from build123d import *

# Parameters (mm, degrees)
SKETCH1_W           = 130
SKETCH1_H           = 82
BOSS_EXTRUDE1_DEPTH = 4
SKETCH2_W           = 40
SKETCH2_H           = 10
CUT_EXTRUDE1_DEPTH  = 24
BOSS_EXTRUDE2_DEPTH = 4
SKETCH4_W           = 10
SKETCH4_H           = 10
BOSS_EXTRUDE3_DEPTH = 24
SKETCH5_R           = 2
CUT_EXTRUDE2_DEPTH  = 151


with BuildPart() as part:
    # Sketch1 → Boss-Extrude1 (new body)
    with BuildSketch(Plane(origin=(0, 0, 0), x_dir=(1, 0, 0), z_dir=(0, 1, 0))):
        Rectangle(SKETCH1_W, SKETCH1_H)
    extrude(amount=BOSS_EXTRUDE1_DEPTH)

    # Sketch2 → Cut-Extrude1 (cut)
    with BuildSketch(Plane(origin=(0, 4, 0), x_dir=(1, 0, 0), z_dir=(0, 1, 0))):
        with Locations((-45, 36)):
            Rectangle(SKETCH2_W, SKETCH2_H)
        with Locations((45, 36)):
            Rectangle(SKETCH2_W, SKETCH2_H)
        with Locations((45, -36)):
            Rectangle(SKETCH2_W, SKETCH2_H)
        with Locations((-45, -36)):
            Rectangle(SKETCH2_W, SKETCH2_H)
    extrude(amount=-CUT_EXTRUDE1_DEPTH, mode=Mode.SUBTRACT)

    # Sketch3 → Boss-Extrude2 (add)
    with BuildSketch(Plane(origin=(0, 4, 0), x_dir=(1, 0, 0), z_dir=(0, 1, 0))):
        Polygon((-65, -31), (-65, 31), (-65, 41), (-75, 41), (-75, -41), (-65, -41), align=None)
        Polygon((75, 41), (65, 41), (65, 31), (65, -31), (65, -41), (75, -41), align=None)
    extrude(amount=-BOSS_EXTRUDE2_DEPTH)

    # Sketch4 → Boss-Extrude3 (add)
    with BuildSketch(Plane(origin=(0, 4, 0), x_dir=(1, 0, 0), z_dir=(0, 1, 0))):
        with Locations((-70, 36)):
            Rectangle(SKETCH4_W, SKETCH4_H)
        with Locations((-20, 36)):
            Rectangle(SKETCH4_W, SKETCH4_H)
        with Locations((20, 36)):
            Rectangle(SKETCH4_W, SKETCH4_H)
        with Locations((70, 36)):
            Rectangle(SKETCH4_W, SKETCH4_H)
        with Locations((70, -36)):
            Rectangle(SKETCH4_W, SKETCH4_H)
        with Locations((20, -36)):
            Rectangle(SKETCH4_W, SKETCH4_H)
        with Locations((-20, -36)):
            Rectangle(SKETCH4_W, SKETCH4_H)
        with Locations((-70, -36)):
            Rectangle(SKETCH4_W, SKETCH4_H)
    extrude(amount=BOSS_EXTRUDE3_DEPTH)

    # Sketch5 → Cut-Extrude2 (cut, through all)
    with BuildSketch(Plane.ZY.offset(75)):
        with Locations((-36, 23)):
            Circle(SKETCH5_R)
        with Locations((36, 23)):
            Circle(SKETCH5_R)
    extrude(amount=-CUT_EXTRUDE2_DEPTH, mode=Mode.SUBTRACT)


solid = part.part
Check sheet for the modelled part. Datum: model origin and axes. Units: mm. A direction names the side the tool comes from. Round coordinates to 2 decimals unless told otherwise and drop trailing zeros. Order: outer loops, then holes, each group sorted by start corner. A loop starts at its lowest first (then second) coordinate and runs counter-clockwise, first axis right, second up.
Q1. Draft check along X on faces 4 (the face through (70, 28, -36)), 5 (the face through (65, 14, 36)), 6 (the face through (75, 3, 0)), 7 (the face through (-75, 3.6, 0.2)). Enter one of: pulls with the +X half, pulls with the -X half, needs draft (parallel to the pull), parting line crosses it, or undercut.
Filled sheet:
face 4: needs draft
face 5: undercut
face 6: pulls with the +X half
face 7: pulls with the -X half
Q2. Cross-section at C-C, the plane x = -9. Enter the section's corners in (y, z).
Filled sheet:
outline: (0, -41) - (4, -41) - (4, 41) - (0, 41) - close
Q3. Set-up check for faces 1 (the face through (45, 2, -31)), 2 (the face through (-70, 16, -31)), 3 (the face through (-70.07, 22.234, 37.847)): record each of +Z, -Z, +X, -X, +Y, -Y from which the full face is reachable in a straight line by a thin tool's end or side.
Filled sheet:
face 1: -Z, +Y, -Y
face 2: +X, -X, +Y
face 3: +X, -X
Q4. Depth check by flat-ended pin: P1, Ø4, axis at x = 0, z = -17, coming from the +Y side; P2, Ø3, axis at y = 18, z = -29, coming from the -X side; P3, Ø2, axis at x = -45, y = 2, coming from the -Z side; P4, Ø4.5, axis at x = 50.5, y = 2.5, coming from the +Z side. Enter the tip coordinate at first touch or a pass-through.
Filled sheet:
P1: stops at y = 4
P2: passes through
P3: stops at z = -31
P4: stops at z = 31
Q5. Cross-section at A-A, the plane y = 8.25. Give the number of separate pieces and of enclosed holes in the cut face, plus the area to 3 significant figures.
Filled sheet:
separate pieces: 8
enclosed holes: 0
area: 800 mm2
Q6. Scan lines: L1, parallel to X at y = 25.5, z = 34; L2, parallel to Y at x = -73, z = 36; L3, parallel to Y at x = 60.5, z = -14. Record each from-to range of solid material in increasing order.
Filled sheet:
L1: x = -75 to -65, -25 to -15, 15 to 25, 65 to 75
L2: y = 0 to 21, 25 to 28
L3: y = 0 to 4
